```python
from build123d import *

# Parameters (mm, degrees)
BOSS_EXTRUDE1_DEPTH = 12.7


with BuildPart() as part:
    # Sketch1 → Boss-Extrude1 (new body)
    with BuildSketch(Plane(origin=(0, 0, 0), x_dir=(0, 0, -1), z_dir=(1, 0, 0))):
        with BuildLine():
            Line((45.172537999, 141.957038049), (11.797012955, 152.577555313))
            ThreePointArc((11.797012955, 152.577555313), (6.406042935, 152.427160627), (2.28061581, 148.95354186))
            ThreePointArc((2.28061581, 148.95354186), (-23.983081912, -147.027788608), (45.172537999, 141.957038049))
        make_face()
        with BuildLine():
            Line((44.787435373, 140.746833121), (11.411910329, 151.367350385))
            ThreePointArc((11.411910329, 151.367350385), (6.525607749, 151.103719143), (3.039474855, 147.669722671))
            ThreePointArc((3.039474855, 147.669722671), (-24.162676495, -145.711188539), (44.787435373, 140.746833121))
        make_face(mode=Mode.SUBTRACT)
    extrude(amount=BOSS_EXTRUDE1_DEPTH)


solid = part.part
```
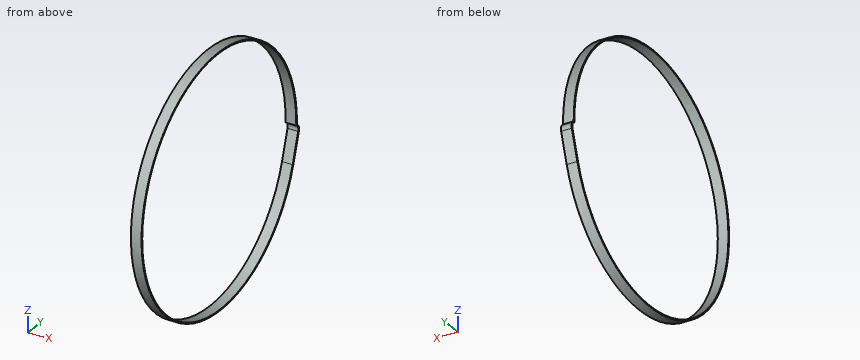
The listing builds one solid part. Answer for the finished solid, in the listing's coordinates (mm). Coordinates: 2 decimals unless noted, no trailing zeros. Loops run counter-clockwise (first coordinate to the right, second up) from the corner with the lowest first, then second, coordinate; pieces in that order, holes last. Notation, with made-up numbers: (-0.75, 42.5) -> (44.25, 42.5) arc R16 cw to (44.25, 64.5) -> close; hole circle Ø3 at (47, -6.5). An arc over 180 degrees is marked (long way). Return JSON: item names as keys, results as strings. Group by question number.
(1) A cutting plane is placed at B-B on x = 7.25. Write down the section's boundary in (y, z).
(2) A cutting plane is placed at A-A on y = 0. Write down the section's boundary in (x, z).
(3) Find the intervals of material crossed by probe 1 along Y at (x, z) = (8.75, 0); probe 2 along Z at (x, y) = (4.5, 91.5), in increasing order. Write a range as from..to.
(4) A cutting plane is placed at C-C on z = -125.5. Write down the section's boundary in (x, y).
(5) Given pin 1 Ø5 at (x, z) = (2, 104) entering from +Y; pin 2 Ø5 at (x, z) = (3, -60) entering from -Y; pin 3 Ø3 at (x, y) = (3, 56) entering from +Z, each flat-ended and moving along its own axis, determine where each tip first touches the part or whether it passes through.
The answers:
{
 "1": {"outline": "(141.96, -45.17) -> (152.58, -11.8) arc R8.18 ccw to (148.95, -2.28) arc R148.97 ccw (long way) to start; hole (140.75, -44.79) -> (151.37, -11.41) arc R6.91 ccw to (147.67, -3.04) arc R147.7 ccw (long way) to start"},
 "2": {"outline": "(0, -148.97) -> (12.7, -148.97) -> (12.7, -147.7) -> (0, -147.7) -> close; (0, 147.7) -> (12.7, 147.7) -> (12.7, 148.97) -> (0, 148.97) -> close"},
 "3": {"probe 1": "y = -148.97..-147.7, 147.7..148.97", "probe 2": "z = -117.56..-115.95, 115.95..117.56"},
 "4": {"outline": "(0, -80.26) -> (12.7, -80.26) -> (12.7, -77.88) -> (0, -77.88) -> close; (0, 77.88) -> (12.7, 77.88) -> (12.7, 80.26) -> (0, 80.26) -> close"},
 "5": {"pin 1": "stops at y = 109.04", "pin 2": "stops at y = -137.43", "pin 3": "stops at z = 138.64"}
}
